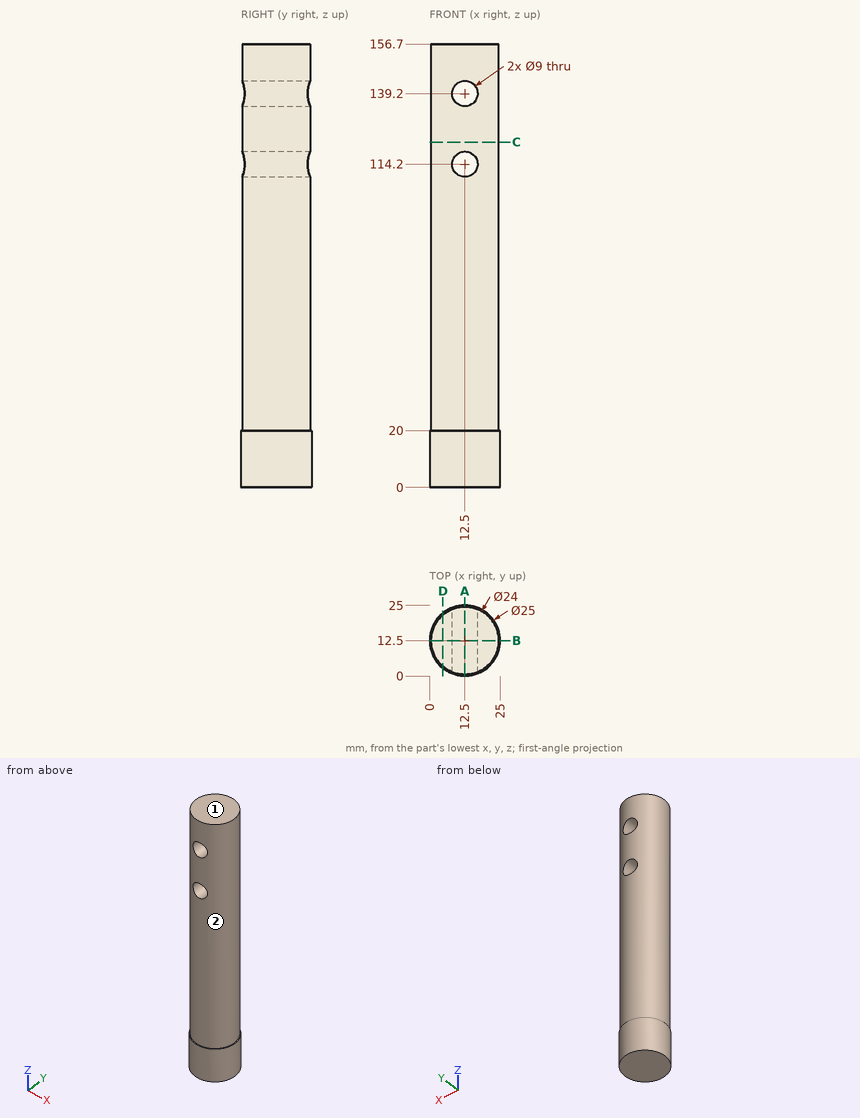
Check sheet for the drawn part. Datum: minimum x, y, z corner. Units: mm. A direction names the side the tool comes from. Round coordinates to 2 decimals unless told otherwise and drop trailing zeros. Loops run counter-clockwise (first coordinate to the right, second up) from the corner with the lowest first, then second, coordinate; pieces in that order, holes last. Notation, with made-up numbers: (15.25, -25) - (67.25, -25) arc R25 ccw to (67.25, -13) - close; hole circle Ø11 at (58.5, 39). An arc over 180 degrees is marked (long way). Write item = value, one per line. Start each with the question number.
1. Section check D-D on x = 4.75. Enter the section's corners in (y, z).
2. Section check B-B on y = 12.5. Enter the section's corners in (x, z).
3. Set-up check for the marked faces 1 and 2: record each of +Z, -Z, +X, -X, +Y, -Y from which the full face is reachable in a straight line by a thin tool's end or side.
4. Depth check by flat-ended pin: pin 1 (1 mm diameter, centred on y = 15, z = 32, fed in from +X); pin 2 (12 mm diameter, centred on x = 6, z = 95.5, fed in from +Y); pin 3 (3 mm diameter, centred on y = 18, z = 40.5, fed in from -X); pin 4 (6 mm diameter, centred on x = 12, y = 22, fed in from -Z). Enter the tip coordinate at first touch or a pass-through.
5. Section check A-A on x = 12.5. Enter the section's corners in (y, z), then the cut area to 3 significant figures.
6. Section check C-C on z = 122. Enter the section's corners in (x, y), then the cut area to 3 significant figures.
7. Thickness scan on line 1 (Z direction, x = 12.5, y = 10.5); line 2 (X direction, y = 12, z = 114.2); line 3 (Z direction, x = 13.75, y = 3). Record the ranges inside material, lowest first.
Working result:
q1.outline = (2.69, 0) - (22.31, 0) - (22.31, 20) - (21.66, 20) - (21.66, 156.7) - (3.34, 156.7) - (3.34, 20) - (2.69, 20) - close
q2.outline = (0, 0) - (25, 0) - (25, 20) - (24.5, 20) - (24.5, 156.7) - (0.5, 156.7) - (0.5, 20) - (0, 20) - close; hole circle Ø9 at (12.5, 114.2); hole circle Ø9 at (12.5, 139.2)
q3.face_1 = +Z, +X, -X, +Y, -Y
q3.face_2 = +Z
q4.pin_1 = 24.33
q4.pin_2 = 24.49
q4.pin_3 = 1.19
q4.pin_4 = 0
q5.outline = (0, 0) - (25, 0) - (25, 20) - (24.5, 20) - (24.5, 109.7) - (0.5, 109.7) - (0.5, 20) - (0, 20) - close; (0.5, 118.7) - (24.5, 118.7) - (24.5, 134.7) - (0.5, 134.7) - close; (0.5, 143.7) - (24.5, 143.7) - (24.5, 156.7) - (0.5, 156.7) - close
q5.area = 3,350 mm^2
q6.outline = circle Ø24 at (12.5, 12.5)
q6.area = 452 mm^2
q7.line_1 = 0 to 109.7, 118.7 to 134.7, 143.7 to 156.7
q7.line_2 = 0.51 to 8, 17 to 24.49
q7.line_3 = 0 to 109.88, 118.52 to 134.88, 143.52 to 156.7
